Can you work these out from the model? Positions are in its coordinate system, mm. Face numbers are marked on the shaded views. Coordinates: 2 decimals unless noted, no trailing zeros. Order: outer loops, then holes, each group sorted by start corner. A loop starts at its lowest first (then second) coordinate and runs counter-clockwise, first axis right, second up. Notation, with made-up numbers: (-19, -4) -> (32, -4) arc R21 cw to (32, 17) -> close; hole circle Ø5 at (1, 85). An arc over 180 degrees is marked (long way). Write item = value, one per line. Start each with the question number.
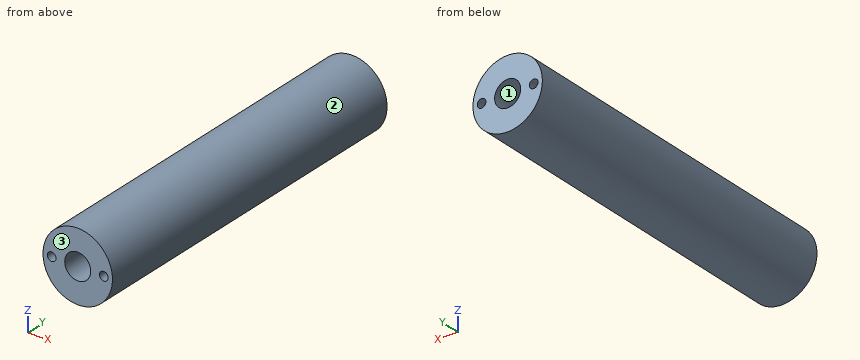
from build123d import *

# Parameters (mm, degrees)
SKETCH1_W               = 12.7
SKETCH1_H               = 259.938138032
SKETCH2_R               = 4.7625
CUT_EXTRUDE1_DEPTH      = 285.124126062
CUT_EXTRUDE2_DEPTH      = 339.459088986
CUT_EXTRUDE2_DEPTH_BACK = 339.459088986
SKETCH3_W               = 82.52004382
SKETCH3_H               = 140.871037148
SKETCH4_R               = 1.5875
CUT_EXTRUDE3_DEPTH      = 12.7
CUT_EXTRUDE4_START      = -12.7
SKETCH5_R               = 1.5875
CUT_EXTRUDE4_DEPTH      = 12.7


with BuildPart() as part:
    # Sketch1 → Revolve1 (revolve)
    with BuildSketch(Plane.XY):
        with Locations((94.956111271, 188.458114984)):
            Rectangle(SKETCH1_W, SKETCH1_H)
    revolve(axis=Axis((101.306111271, 318.427184, 0), (0, -1, 0)))

    # Sketch2 → Cut-Extrude1 (cut, through all)
    with BuildSketch(Plane(origin=(0, 318.427184, 0), x_dir=(1, 0, 0), z_dir=(0, 1, 0))):
        with Locations(Location((101.306111271, 0, 0), (0, 0, 180))):
            Circle(SKETCH2_R)
    extrude(amount=-CUT_EXTRUDE1_DEPTH, mode=Mode.SUBTRACT)

    # Sketch3 → Cut-Extrude2 (cut, two sides: drawn at the far end of the back side and taken through both)
    with BuildSketch(Plane.XY.offset(-CUT_EXTRUDE2_DEPTH_BACK)):
        with Locations((93.882760048, 258.893633558)):
            Rectangle(SKETCH3_W, SKETCH3_H)
    extrude(amount=CUT_EXTRUDE2_DEPTH + CUT_EXTRUDE2_DEPTH_BACK, mode=Mode.SUBTRACT)

    # Sketch4 → Cut-Extrude3 (cut)
    with BuildSketch(Plane(origin=(0, 188.458114984, 0), x_dir=(1, 0, 0), z_dir=(0, 1, 0))):
        with Locations(Location((91.781111271, 0, 0), (0, 0, 270))):
            Circle(SKETCH4_R)
        with Locations(Location((110.831111271, 0, 0), (0, 0, 270))):
            Circle(SKETCH4_R)
    extrude(amount=-CUT_EXTRUDE3_DEPTH, mode=Mode.SUBTRACT)

    # Sketch5 → Cut-Extrude4 (cut)
    with BuildSketch(Plane.XZ.offset(-58.489045968).offset(CUT_EXTRUDE4_START)):
        with Locations(Location((91.781111271, 0, 0), (0, 0, 90))):
            Circle(SKETCH5_R)
        with Locations(Location((110.831111271, 0, 0), (0, 0, 90))):
            Circle(SKETCH5_R)
    extrude(amount=CUT_EXTRUDE4_DEPTH, mode=Mode.SUBTRACT)


solid = part.part
(1) Imagine slicing it at A-A (z = 0). Write out the boundary of the cut face in (x, y), plus the area to 3 significant figures.
(2) Imagine slicing it at C-C (x = 100). Write out the boundary of the cut face in (y, z), plus the area to 3 significant figures.
(3) If I drill on L1, parallel to Z at x = 101, y = 136.5; L2, parallel to X at y = 121, z = 0.5; L3, parallel to X at y = 124, z = 2.5, over which ranges is the centre line in solid material (lowest first)? Write a range as from..to.
(4) For P1, Ø1, axis at y = 101, z = 5.5, coming from the -X side; P2, Ø1.9, axis at x = 110.83, z = 0, coming from the -Y side; P3, Ø5, axis at y = 145, z = 8, coming from the +X side, each with a flat end and sliding along its axis, tell me the tip position at first contact or that it passes through.
(5) Thinking about a two-plate mould opening in Z: for the marked faces 1, 2 and 3, which applies, +Z half, -Z half, draft (parallel to the pull), parting line (faces both ways), or undercut?
(6) Imagine slicing it at D-D (z = -8.25). Write out the boundary of the cut face in (x, y), plus the area to 3 significant figures.
(7) Imagine slicing it at B-B (y = 93.5). Write out the boundary of the cut face in (x, z) (1 decimal), plus the area to 3 significant figures.
Result set:
q1.outline = (88.61, 58.49) -> (90.19, 58.49) -> (90.19, 71.19) -> (93.37, 71.19) -> (93.37, 58.49) -> (96.54, 58.49) -> (96.54, 188.46) -> (93.37, 188.46) -> (93.37, 175.76) -> (90.19, 175.76) -> (90.19, 188.46) -> (88.61, 188.46) -> close; (106.07, 58.49) -> (109.24, 58.49) -> (109.24, 71.19) -> (112.42, 71.19) -> (112.42, 58.49) -> (114.01, 58.49) -> (114.01, 188.46) -> (112.42, 188.46) -> (112.42, 175.76) -> (109.24, 175.76) -> (109.24, 188.46) -> (106.07, 188.46) -> close
q1.area = 1,900 mm2
q2.outline = (58.49, -12.63) -> (188.46, -12.63) -> (188.46, -4.58) -> (58.49, -4.58) -> close; (58.49, 4.58) -> (188.46, 4.58) -> (188.46, 12.63) -> (58.49, 12.63) -> close
q2.area = 2,090 mm2
q3.L1 = -12.7..-4.75, 4.75..12.7
q3.L2 = 88.62..96.57, 106.04..114
q3.L3 = 88.85..97.25, 105.36..113.76
q4.P1 = 89.63
q4.P2 = 71.19
q4.P3 = 112.75
q5.face_1 = undercut
q5.face_2 = parting line
q5.face_3 = draft
q6.outline = (91.65, 58.49) -> (110.96, 58.49) -> (110.96, 188.46) -> (91.65, 188.46) -> close
q6.area = 2,510 mm2
q7.outline = circle Ø25.4 at (101.3, 0); hole circle Ø9.5 at (101.3, 0)
q7.area = 435 mm2
